Design review of the part built by this model. Coordinates are the model's own, in mm. Face numbers are marked on the shaded views. A direction names the side the tool comes from. Give positions to 0.01 mm unless a question says otherwise; leave off trailing zeros. Order: outer loops, then holes, each group sorted by start corner. A loop starts at its lowest first (then second) coordinate and runs counter-clockwise, first axis right, second up. Notation, with made-up numbers: (26.25, -2) -> (69.25, -2) arc R13 cw to (69.25, 18) -> close; hole circle Ø7 at (35, 39.25). An arc over 180 degrees is marked (long way). Return JSON: item names as keys, results as strings.
```python
from build123d import *

# Parameters (mm, degrees)
BOSS_EXTRUDE1_DEPTH = 50.8
SKETCH3_R           = 11.1
CUT_EXTRUDE1_DEPTH  = 6
SKETCH4_R           = 9.6
CUT_EXTRUDE2_DEPTH  = 87.597575024
CUT_EXTRUDE3_DEPTH  = 84.529276305
FILLET1_R           = 20
FILLET2_R           = 12
SKETCH6_R           = 3
CUT_EXTRUDE4_DEPTH  = 89.809571556
SKETCH7_W           = 28.5
SKETCH7_H           = 30.8
CUT_EXTRUDE5_DEPTH  = 85.592493757
FILLET3_R           = 6
FILLET4_R           = 6
FILLET5_R           = 12
CHAMFER1_SIZE       = 0.5
CHAMFER2_SIZE       = 1


with BuildPart() as part:
    # Sketch2 → Boss-Extrude1 (new body)
    with BuildSketch(Plane(origin=(0, 0, 0), x_dir=(1, 0, 0), z_dir=(0, 1, 0))):
        Polygon((0, 7.5), (50.5, 7.5), (50.5, -52.5), (40.5, -52.5), (40.5, -7.5), (0, -7.5), align=None)
    extrude(amount=BOSS_EXTRUDE1_DEPTH)

    # Sketch3 → Cut-Extrude1 (cut)
    with BuildSketch(Plane.ZY.offset(-40.5)):
        with Locations((38.5, 35.4)):
            Circle(SKETCH3_R)
    extrude(amount=-CUT_EXTRUDE1_DEPTH, mode=Mode.SUBTRACT)

    # Sketch4 → Cut-Extrude2 (cut, through all)
    with BuildSketch(Plane.ZY.offset(-46.5)):
        with Locations((38.5, 35.4)):
            Circle(SKETCH4_R)
    extrude(amount=-CUT_EXTRUDE2_DEPTH, mode=Mode.SUBTRACT)

    # Sketch5 → Cut-Extrude3 (cut, through all)
    with BuildSketch(Plane.ZY.offset(-40.5)):
        Polygon((12.5, 0), (52.5, 0), (52.5, 26), align=None)
    extrude(amount=-CUT_EXTRUDE3_DEPTH, mode=Mode.SUBTRACT)

    # Fillet1
    fillet1_edges = [part.edges().sort_by_distance(p)[0] for p in [
        (45.5, 26, 52.5),
    ]]
    fillet(fillet1_edges, radius=FILLET1_R)

    # Fillet2
    fillet2_edges = [part.edges().sort_by_distance(p)[0] for p in [
        (45.5, 50.8, 52.5),
    ]]
    fillet(fillet2_edges, radius=FILLET2_R)

    # Sketch6 → Cut-Extrude4 (cut, through all)
    with BuildSketch(Plane(origin=(0, 50.8, 0), x_dir=(1, 0, 0), z_dir=(0, 1, 0))):
        with Locations(Location((6, 0, 0), (0, 0, 270))):
            Circle(SKETCH6_R)
        with Locations(Location((32, 0, 0), (0, 0, 270))):
            Circle(SKETCH6_R)
    extrude(amount=-CUT_EXTRUDE4_DEPTH, mode=Mode.SUBTRACT)

    # Sketch7 → Cut-Extrude5 (cut, through all)
    with BuildSketch(Plane.XY.offset(7.5)):
        with Locations((14.25, 25.4)):
            Rectangle(SKETCH7_W, SKETCH7_H)
    extrude(amount=-CUT_EXTRUDE5_DEPTH, mode=Mode.SUBTRACT)

    # Fillet3
    fillet3_edges = [part.edges().sort_by_distance(p)[0] for p in [
        (28.5, 10, 0),
        (28.5, 40.8, 0),
    ]]
    fillet(fillet3_edges, radius=FILLET3_R)

    # Fillet4
    fillet4_edges = [part.edges().sort_by_distance(p)[0] for p in [
        (50.5, 25.4, -7.5),
    ]]
    fillet(fillet4_edges, radius=FILLET4_R)

    # Fillet5
    fillet5_edges = [part.edges().sort_by_distance(p)[0] for p in [
        (45.5, 0, 12.5),
    ]]
    fillet(fillet5_edges, radius=FILLET5_R)

    # Chamfer1
    chamfer1_edges = [part.edges().sort_by_distance(p)[0] for p in [
        (48.742640687, 0, -5.742640687),
        (50.5, 50.8, 19.5),
        (48.742640687, 50.8, -5.742640687),
        (40.5, 0, 8.221359592),
        (40.5, 0.4948733, 12.353299725),
        (50.5, 0.4948733, 12.353299725),
        (0, 45.8, -7.5),
        (0, 45.8, 7.5),
        (20.25, 50.8, 7.5),
        (0, 50.8, 0),
        (40.5, 11.011762581, 29.441173202),
        (50.5, 11.011762581, 29.441173202),
        (40.5, 27.314206751, 50.07832956),
        (50.5, 27.314206751, 50.07832956),
        (40.5, 37.826860442, 52.5),
        (50.5, 37.826860442, 52.5),
        (40.5, 50.8, 24),
        (22.25, 50.8, -7.5),
        (40.5, 47.285281374, 48.985281374),
        (50.5, 47.285281374, 48.985281374),
        (0, 5, 7.5),
        (0, 0, 0),
        (0, 5, -7.5),
        (20.25, 0, 7.5),
        (0, 40.8, 0),
        (11.25, 10, -7.5),
        (0, 10, 0),
        (11.25, 10, 7.5),
        (11.25, 40.8, 7.5),
        (11.25, 40.8, -7.5),
        (28.5, 25.4, 7.5),
        (28.5, 25.4, -7.5),
        (22.25, 0, -7.5),
        (26.742640687, 39.042640687, 7.5),
        (26.742640687, 39.042640687, -7.5),
        (26.742640687, 11.757359313, 7.5),
        (26.742640687, 11.757359313, -7.5),
        (50.5, 0, 3.721359592),
    ]]
    chamfer(chamfer1_edges, length=CHAMFER1_SIZE)

    # Chamfer2
    chamfer2_edges = [part.edges().sort_by_distance(p)[0] for p in [
        (40.5, 35.4, 27.4),
    ]]
    chamfer(chamfer2_edges, length=CHAMFER2_SIZE)


solid = part.part
```
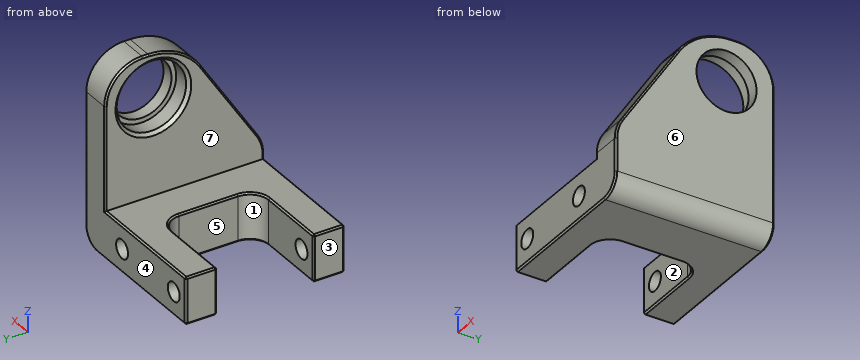
Item 1: Add section B-B (z = 0). Give the boundary of the cut face in (x, y), plus the area to 3 significant figures.
Result set:
{"outline": "(0, 0.5) -> (0.5, 0) -> (3, 0) -> (3, 10) -> (0.5, 10) -> (0, 9.5) -> close; (0, 41.3) -> (0.5, 40.8) -> (3, 40.8) -> (3, 50.8) -> (0.5, 50.8) -> (0, 50.3) -> close; (9, 0) -> (29, 0) -> (29, 50.8) -> (9, 50.8) -> (9, 40.8) -> (22.5, 40.8) arc R6 cw to (28.5, 34.8) -> (28.5, 16) arc R6 cw to (22.5, 10) -> (9, 10) -> close; (35, 0) -> (50, 0) -> (50.5, 0.5) -> (50.5, 50.3) -> (50, 50.8) -> (35, 50.8) -> close", "area": "1,280 mm^2"}
Item 2: Mouldability with a two-part tool opening along Y and no side actions: class the marked faces 1, 2, 3 and 4 as released by +Y, released by -Y, zero draft, split by the parting line, or undercut.
Result set:
{"face 1": "undercut", "face 2": "undercut", "face 3": "zero draft", "face 4": "released by +Y"}
Item 3: Wall thickness on L1, parallel to X at y = 48, z = 0; L2, parallel to X at y = 21, z = 0; L3, parallel to Z at x = 42.5, y = 26: over which ranges is each line inside the solid? List them lowest first. Write a range as [from, to].
Result set:
{"L1": "x = [0, 3], [9, 29], [35, 50.5]", "L2": "x = [28.5, 29], [35, 50.5]", "L3": "z = [-7.5, 32.6], [44.4, 49.3]"}
Item 4: Machinability: for the marked faces 5, 6 and 7, which of the approach directions +Z, -Z, +X, -X, +Y, -Y give a long, thin tool a straight path to every point of the face, cutting with its end or side? Answer none if there is none.
Result set:
{"face 5": "+Z, -Z, -X", "face 6": "+Z, -Z, +X, +Y, -Y", "face 7": "+Z, -X, +Y, -Y"}
Item 5: Add section A-A (x = 32). Give the boundary of the cut face in (y, z).
Result set:
{"outline": "(0, -7) -> (0.5, -7.5) -> (50.3, -7.5) -> (50.8, -7) -> (50.8, -3) -> (0, -3) -> close; (0, 3) -> (50.8, 3) -> (50.8, 7) -> (50.3, 7.5) -> (0.5, 7.5) -> (0, 7) -> close"}
Item 6: Add section D-D (x = 43). Give the boundary of the cut face in (y, z), plus the area to 3 significant figures.
Result set:
{"outline": "(0, -7) -> (0.5, -7.5) -> (50.3, -7.5) -> (50.8, -7) -> (50.8, 40.5) arc R12 ccw to (38.8, 52.5) -> (36.85, 52.5) arc R20 ccw to (20.08, 43.4) -> (1.94, 15.48) arc R12 ccw to (0, 8.94) -> close; hole circle Ø22.2 at (35.4, 38.5)", "area": "2,090 mm^2"}
Item 7: Add section C-C (x = 6). Give the boundary of the cut face in (y, z).
Result set:
{"outline": "(0, -7) -> (0.5, -7.5) -> (9.5, -7.5) -> (10, -7) -> (10, -3) -> (0, -3) -> close; (0, 3) -> (10, 3) -> (10, 7) -> (9.5, 7.5) -> (0.5, 7.5) -> (0, 7) -> close; (40.8, -7) -> (41.3, -7.5) -> (50.3, -7.5) -> (50.8, -7) -> (50.8, -3) -> (40.8, -3) -> close; (40.8, 3) -> (50.8, 3) -> (50.8, 7) -> (50.3, 7.5) -> (41.3, 7.5) -> (40.8, 7) -> close"}
Item 8: For pin 1 (7 mm diameter, centred on y = 21.5, z = -1.5, fed in from -X); pin 2 (20 mm diameter, centred on x = 15.5, y = 13.5, fed in from +Z); pin 3 (8 mm diameter, centred on x = 40.5, y = 19.5, fed in from +Z), all flat-tipped, find the tip position at first contact; note any pin that passes through.
Result set:
{"pin 1": "stops at x = 28.5", "pin 2": "stops at z = 7.5", "pin 3": "stops at z = 47.36"}
